from build123d import *

# Parameters (mm, degrees)
F0_R     = 12.7
F1_DEPTH = 12.7
F2_R     = 4.7625
F3_DEPTH = 9.652
F5_DEPTH = 9.525
F6_R     = 1.5875
F7_DEPTH = 6.35


with BuildPart() as f1:
    # F0 (on Front) → F1 (new body)
    with BuildSketch(Plane.XZ):
        Circle(F0_R)
    extrude(amount=F1_DEPTH)

    # F2 (on face) → F3 (join)
    with BuildSketch(Plane.XZ.offset(12.7)):
        Circle(F2_R)
    extrude(amount=F3_DEPTH)

    # F4 (on face) → F5 (cut)
    with BuildSketch(Plane.XZ.offset(22.352)):
        with BuildLine():
            ThreePointArc((1.5875, 4.490128), (0, 4.7625), (-1.5875, 4.490128))
            Line((-1.5875, 4.490128), (-1.5875, -4.490128))
            ThreePointArc((-1.5875, -4.490128), (0, -4.7625), (1.5875, -4.490128))
            Line((1.5875, -4.490128), (1.5875, 4.490128))
        make_face()
    extrude(amount=-F5_DEPTH, mode=Mode.SUBTRACT)

    # F6 (on face) → F7 (cut, symmetric)
    with BuildSketch(Plane.YZ.offset(-1.5875)):
        with Locations((-19.177, 0)):
            Circle(F6_R)
    extrude(amount=F7_DEPTH, both=True, mode=Mode.SUBTRACT)


solid = f1.part
For this review, take the finished solid that the model builds, in its own axes (mm). A direction names the side the tool comes from. Round coordinates to 2 decimals unless told otherwise and drop trailing zeros. Write each loop counter-clockwise with the first axis right and the second up, starting at its lowest first coordinate (ties: lowest second). Pieces come first, ordered by that corner, then holes. Notation, with made-up numbers: (35, -4) - (58, -4) arc R12 cw to (58, 2) - close; hole circle Ø8 at (46, -34). An arc over 180 degrees is marked (long way). Use a Markdown table: item, result.
Q1. We need section A-A (z = 0). Give the boundary of the cut face in (x, y).
Derived:
| item | result |
|---|---|
| outline | (-12.7, -12.7) - (-4.76, -12.7) - (-4.76, -17.59) - (-1.59, -17.59) - (-1.59, -12.83) - (1.59, -12.83) - (1.59, -17.59) - (4.76, -17.59) - (4.76, -12.7) - (12.7, -12.7) - (12.7, 0) - (-12.7, 0) - close; (-4.76, -22.35) - (-1.59, -22.35) - (-1.59, -20.76) - (-4.76, -20.76) - close; (1.59, -22.35) - (4.76, -22.35) - (4.76, -20.76) - (1.59, -20.76) - close |
Q2. We need section C-C (x = 0). Give the boundary of the cut face in (y, z).
Derived:
| item | result |
|---|---|
| outline | (-12.83, -4.76) - (-12.7, -4.76) - (-12.7, -12.7) - (0, -12.7) - (0, 12.7) - (-12.7, 12.7) - (-12.7, 4.76) - (-12.83, 4.76) - close |
Q3. Clearance check with flat-ended pins moving along their axes: pin 1 (12 mm diameter, centred on x = -6.5, y = -19.5, fed in from -Z); pin 2 (4.5 mm diameter, centred on y = -15.5, z = 0.5, fed in from -X); pin 3 (1 mm diameter, centred on x = -0.5, z = 1, fed in from -Y). State where each tip first meets the part, or that it passes through.
Derived:
| item | result |
|---|---|
| pin 1 | stops at z = -4.49 |
| pin 2 | stops at x = -4.76 |
| pin 3 | stops at y = -12.83 |
Q4. Machinability: for faces 1 (the flat face through (5, -12.7, 0)), 2 (the cylindrical face through (3.197, -20.763, 0.07)), 3 (the flat face through (-1.588, -17, 0)), which of the approach directions +Z, -Z, +X, -X, +Y, -Y give a long, thin tool a straight path to every point of the face, cutting with its end or side? Answer none if there is none.
Derived:
| item | result |
|---|---|
| face 1 | -Y |
| face 2 | +X, -X |
| face 3 | +Z, -Z, -Y |
Q5. We need section B-B (y = -13.5). Give the boundary of the cut face in (x, z) (1 decimal).
Derived:
| item | result |
|---|---|
| outline | (-1.6, -4.5) - (-1.6, 4.5) arc R4.8 ccw to start; (1.6, -4.5) arc R4.8 ccw to (1.6, 4.5) - close |
Q6. We need section D-D (x = -3.5). Give the boundary of the cut face in (y, z) (1 decimal), plus the area to 3 significant figures.
Derived:
| item | result |
|---|---|
| outline | (-22.4, -3.2) - (-12.7, -3.2) - (-12.7, -12.2) - (0, -12.2) - (0, 12.2) - (-12.7, 12.2) - (-12.7, 3.2) - (-22.4, 3.2) - close; hole circle Ø3.2 at (-19.2, 0) |
| area | 365 mm2 |
Q7. Wall thickness on line 1 along Y through (x, z) = (2.9, 0); line 2 along Y through (x, z) = (-7.5, -5.5); line 3 along Z through (x, y) = (-0.25, -9.75): over which ranges is each line inside the solid? List them lowest first.
Derived:
| item | result |
|---|---|
| line 1 | y = -22.35 to -20.76, -17.59 to 0 |
| line 2 | y = -12.7 to 0 |
| line 3 | z = -12.7 to 12.7 |
Q8. The part is to be moulded in two halves that separate along X. For faces 4 (the cylindrical face through (-2.75, -6.26, -12.4)), 5 (the flat face through (0, -12.827, 0)), 6 (the flat face through (0, 0, 0)), say which applies: pulls with the +X half, pulls with the -X half, needs draft (parallel to the pull), parting line crosses it, or undercut.
Derived:
| item | result |
|---|---|
| face 4 | parting line crosses it |
| face 5 | undercut |
| face 6 | needs draft |
